```python
from build123d import *

# Parameters (mm, degrees)
SKETCH1_R           = 76.2
BOSS_EXTRUDE1_DEPTH = 6.35
SKETCH2_R           = 1.905
CUT_EXTRUDE1_DEPTH  = 108.95
SKETCH3_R           = 3.429
CUT_EXTRUDE2_DEPTH  = 108.95
SKETCH4_R           = 3.429
CUT_EXTRUDE3_DEPTH  = 108.95
SKETCH5_R           = 2.54
CUT_EXTRUDE4_DEPTH  = 108.95
CUT_EXTRUDE5_DEPTH  = 108.95


with BuildPart() as part:
    # Sketch1 → Boss-Extrude1 (new body)
    with BuildSketch(Plane(origin=(0, 0, 0), x_dir=(1, 0, 0), z_dir=(0, 1, 0))):
        with Locations(Location((0, 0, 0), (0, 0, 270))):
            Circle(SKETCH1_R)
    extrude(amount=BOSS_EXTRUDE1_DEPTH)

    # Sketch2 → Cut-Extrude1 (cut, through all)
    with BuildSketch(Plane(origin=(0, 6.35, 0), x_dir=(1, 0, 0), z_dir=(0, 1, 0))):
        with Locations(Location((0, 0, 0), (0, 0, 270))):
            Circle(SKETCH2_R)
    extrude(amount=-CUT_EXTRUDE1_DEPTH, mode=Mode.SUBTRACT)

    # Sketch3 → Cut-Extrude2 (cut, through all)
    with BuildSketch(Plane(origin=(0, 6.35, 0), x_dir=(1, 0, 0), z_dir=(0, 1, 0))):
        with Locations(Location((0, 14.732, 0), (0, 0, 270))):
            Circle(SKETCH3_R)
        with Locations(Location((-13.97, -10.631143259, 0), (0, 0, 270))):
            Circle(SKETCH3_R)
        with Locations(Location((13.97, -10.631143259, 0), (0, 0, 270))):
            Circle(SKETCH3_R)
    extrude(amount=-CUT_EXTRUDE2_DEPTH, mode=Mode.SUBTRACT)

    # Sketch4 → Cut-Extrude3 (cut, through all)
    with BuildSketch(Plane(origin=(0, 6.35, 0), x_dir=(1, 0, 0), z_dir=(0, 1, 0))):
        with Locations(Location((-57.15, 0, 0), (0, 0, 270))):
            Circle(SKETCH4_R)
        with Locations(Location((48.26, 31.75, 0), (0, 0, 270))):
            Circle(SKETCH4_R)
        with Locations(Location((48.26, -31.75, 0), (0, 0, 270))):
            Circle(SKETCH4_R)
    extrude(amount=-CUT_EXTRUDE3_DEPTH, mode=Mode.SUBTRACT)

    # Sketch5 → Cut-Extrude4 (cut, through all)
    with BuildSketch(Plane(origin=(0, 6.35, 0), x_dir=(1, 0, 0), z_dir=(0, 1, 0))):
        with Locations(Location((0, 55.88, 0), (0, 0, 270))):
            Circle(SKETCH5_R)
    extrude(amount=-CUT_EXTRUDE4_DEPTH, mode=Mode.SUBTRACT)

    # Sketch6 → Cut-Extrude5 (cut, through all)
    with BuildSketch(Plane(origin=(0, 6.35, 0), x_dir=(1, 0, 0), z_dir=(0, 1, 0))):
        with BuildLine():
            ThreePointArc((-13.024260998, -27.814715677), (-13.342299809, -26.651562737), (-14.207922206, -25.812056148))
            Line((-14.207922206, -25.812056148), (-16.412599789, -29.817375206))
            ThreePointArc((-16.412599789, -29.817375206), (-14.147108058, -29.782676865), (-13.024260998, -27.814715677))
        make_face()
        with BuildLine():
            Line((-16.412599789, -29.817375206), (-14.207922206, -25.812056148))
            ThreePointArc((-14.207922206, -25.812056148), (-17.312920526, -26.712376885), (-16.412599789, -29.817375206))
        make_face()
        with BuildLine():
            ThreePointArc((17.596260998, 27.814715677), (17.278222186, 28.977868616), (16.412599789, 29.817375206))
            Line((16.412599789, 29.817375206), (14.207922206, 25.812056148))
            ThreePointArc((14.207922206, 25.812056148), (16.473413937, 25.846754488), (17.596260998, 27.814715677))
        make_face()
        with BuildLine():
            Line((14.207922206, 25.812056148), (16.412599789, 29.817375206))
            ThreePointArc((16.412599789, 29.817375206), (13.307601469, 28.917054469), (14.207922206, 25.812056148))
        make_face()
    extrude(amount=-CUT_EXTRUDE5_DEPTH, mode=Mode.SUBTRACT)


solid = part.part
```
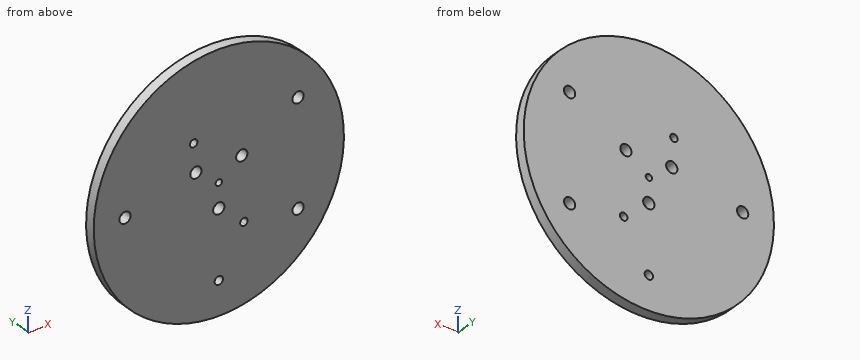
CAD build for the part. Positions are in the model's coordinates, mm. Round coordinates to 2 decimals unless told otherwise and drop trailing zeros. Order: outer loops, then holes, each group sorted by start corner. A loop starts at its lowest first (then second) coordinate and runs counter-clockwise, first axis right, second up.
Item 1: Saw through at B-B on y = 2.75. State how many separate pieces and enclosed holes the cut face has, then the cut area to 3 significant figures.
Item 2: Probe line 1 along X through (y, z) = (2.5, 0) (3 decimals); line 2 along X through (y, z) = (4, -0.5); line 3 along Z through (x, y) = (-2, 3.5). List the from-to ranges inside material, lowest first.
Item 3: Saw through at D-D on z = -16. Write the cut outline in (x, y).
Item 4: Pin check, flat tips, straight feed: pin 1 (3 mm diameter, centred on y = 3.5, z = -22, fed in from +X); pin 2 (5 mm diameter, centred on x = 53, z = -36.5, fed in from -Y); pin 3 (2 mm diameter, centred on y = 5, z = 8, fed in from +X); pin 4 (3 mm diameter, centred on x = 2, y = 2, fed in from +Z). Stop position of each tip, or through.
Item 5: Saw through at A-A on x = 0. Write the cut outline in (y, z) (3 decimals).
Item 6: Saw through at C-C on z = 0. Write the cut outline in (x, y) (3 decimals).
Reported:
1. separate pieces: 1
1. enclosed holes: 10
1. area: 18,000 mm2
2. line 1: x = -76.2 to -60.579, -53.721 to -1.905, 1.905 to 76.2
2. line 2: x = -76.2 to -60.54, -53.76 to -1.84, 1.84 to 76.2
2. line 3: z = -76.17 to -57.45, -54.31 to -17.52, -11.95 to 76.17
3. outline: (-74.5, 0) - (-3.19, 0) - (-3.19, 6.35) - (-74.5, 6.35) - close; (3.19, 0) - (74.5, 0) - (74.5, 6.35) - (3.19, 6.35) - close
4. pin 1: stops at x = 73.39
4. pin 2: stops at y = 0
4. pin 3: stops at x = 75.88
4. pin 4: stops at z = 76.2
5. outline: (0, -76.2) - (6.35, -76.2) - (6.35, -58.42) - (0, -58.42) - close; (0, -53.34) - (6.35, -53.34) - (6.35, -18.161) - (0, -18.161) - close; (0, -11.303) - (6.35, -11.303) - (6.35, -1.905) - (0, -1.905) - close; (0, 1.905) - (6.35, 1.905) - (6.35, 76.2) - (0, 76.2) - close
6. outline: (-76.2, 0) - (-60.579, 0) - (-60.579, 6.35) - (-76.2, 6.35) - close; (-53.721, 0) - (-1.905, 0) - (-1.905, 6.35) - (-53.721, 6.35) - close; (1.905, 0) - (76.2, 0) - (76.2, 6.35) - (1.905, 6.35) - close
